Could you check a few things on this drawing? It's one solid part, dimensions in mm from its lowest x, y, z. A direction names the side the tool comes from. Give positions to 0.01 mm unless a question says otherwise; leave off trailing zeros. Order: outer loops, then holes, each group sorted by start corner. A loop starts at its lowest first (then second) coordinate and runs counter-clockwise, first axis right, second up. Notation, with made-up numbers: (56, -34) - (94, -34) arc R24 cw to (94, -24) - close; hole circle Ø2 at (-9.75, 32). An arc over 180 degrees is marked (long way). One line per question, with ' | ' between items. Start each with the question number.
1. Imagine slicing it at C-C (x = 110). Please give me the cut outline in (y, z), and give its area (3 significant figures).
2. Imagine slicing it at D-D (z = 38). Please give me the cut outline in (x, y), and give its area (3 significant figures).
3. Imagine slicing it at A-A (x = 130). Please give me the cut outline in (y, z).
4. For P1, Ø5, axis at x = 77, y = 10, coming from the -Z side; P2, Ø0.8, axis at x = 6, y = 51, coming from the +Z side; P3, Ø12.5, axis at y = 19, z = 39, coming from the +X side, each with a flat end and sliding along its axis, tell me the tip position at first contact or that it passes through.
5. Which directions (+Z, -Z, +X, -X, +Y, -Y) give clear straight access to the entire face, cutting with the end or side of a thin tool? Please do the marked faces 1 and 2.
6. Imagine slicing it at B-B (z = 10). Please give me the cut outline in (x, y), and give its area (3 significant figures).
7. I need wall thicknesses on probe 1 along X at (y, z) = (50.5, 10); probe 2 along Z at (x, y) = (130, 51); probe 3 along Y at (x, z) = (54, 12). Which ranges of each line are inside material? Lowest first, please. Write a range as from..to.
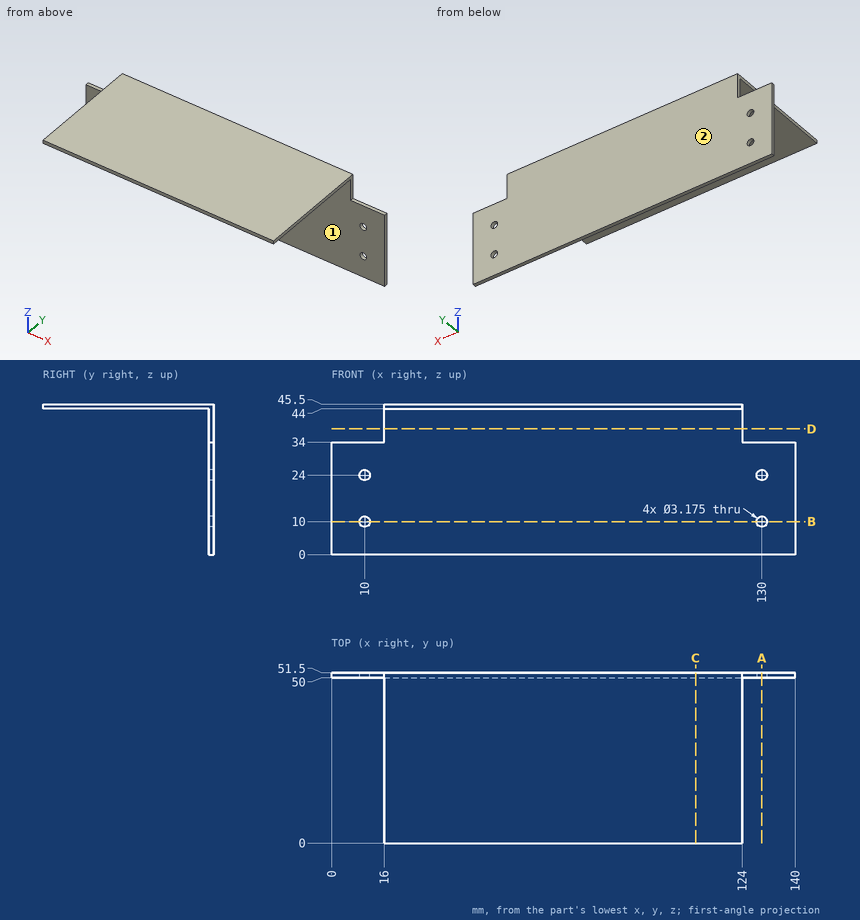
Results found:
1) outline: (0, 44) - (50, 44) - (50, 0) - (51.5, 0) - (51.5, 45.5) - (0, 45.5) - close | area: 143 mm2
2) outline: (16, 50) - (124, 50) - (124, 51.5) - (16, 51.5) - close | area: 162 mm2
3) outline: (50, 0) - (51.5, 0) - (51.5, 8.41) - (50, 8.41) - close; (50, 11.59) - (51.5, 11.59) - (51.5, 22.41) - (50, 22.41) - close; (50, 25.59) - (51.5, 25.59) - (51.5, 34) - (50, 34) - close
4) P1: stops at z = 44 | P2: stops at z = 34 | P3: stops at x = 124
5) face 1: -Z, +X, -X, -Y | face 2: +Z, -Z, +X, -X, +Y
6) outline: (0, 50) - (8.41, 50) - (8.41, 51.5) - (0, 51.5) - close; (11.59, 50) - (128.41, 50) - (128.41, 51.5) - (11.59, 51.5) - close; (131.59, 50) - (140, 50) - (140, 51.5) - (131.59, 51.5) - close | area: 200 mm2
7) probe 1: x = 0..8.41, 11.59..128.41, 131.59..140 | probe 2: z = 0..8.41, 11.59..22.41, 25.59..34 | probe 3: y = 50..51.5
